Read the model definition and answer for the solid it produces. Units are mm, in the model's axes. A direction names the side the tool comes from. Round coordinates to 2 decimals unless told otherwise and drop trailing zeros. Order: outer loops, then holes, each group sorted by start corner. A loop starts at its lowest first (then second) coordinate and runs counter-clockwise, first axis right, second up.
from build123d import *

# Parameters (mm, degrees)
SKETCH1_R                                         = 8
BOSS_EXTRUDE1_DEPTH                               = 30
SKETCH2_R                                         = 1.5
CUT_EXTRUDE2_DEPTH                                = 30
CSK_FOR_2_FLAT_HEAD_MACHINE_SCREW_100_D           = 2.7051
CSK_FOR_2_FLAT_HEAD_MACHINE_SCREW_100_CSINK_D     = 4.3688
CSK_FOR_2_FLAT_HEAD_MACHINE_SCREW_100_CSINK_ANGLE = 100
CSK_FOR_2_FLAT_HEAD_MACHINE_SCREW_2_D             = 2.7051
CSK_FOR_2_FLAT_HEAD_MACHINE_SCREW_2_CSINK_D       = 4.3688
CSK_FOR_2_FLAT_HEAD_MACHINE_SCREW_2_CSINK_ANGLE   = 100
CSK_FOR_2_FLAT_HEAD_MACHINE_SCREW_3_D             = 2.7051
CSK_FOR_2_FLAT_HEAD_MACHINE_SCREW_3_CSINK_D       = 4.3688
CSK_FOR_2_FLAT_HEAD_MACHINE_SCREW_3_CSINK_ANGLE   = 100
CSK_FOR_2_FLAT_HEAD_MACHINE_SCREW_4_D             = 2.7051
CSK_FOR_2_FLAT_HEAD_MACHINE_SCREW_4_CSINK_D       = 4.3688
CSK_FOR_2_FLAT_HEAD_MACHINE_SCREW_4_CSINK_ANGLE   = 100


with BuildPart() as part:
    # Sketch1 → Boss-Extrude1 (new body)
    with BuildSketch(Plane.XY):
        Polygon((33.27, 7), (31.19936412, 7), (31.19936412, 17), (23.19936412, 17), (19.69936412, 22.18), (13.57063588, 22.18), (10.07063588, 17), (2.07063588, 17), (2.07063588, 7), (0, 7), (0, 0), (33.27, 0), align=None)
        with Locations((16.635, 10.68)):
            Circle(SKETCH1_R, mode=Mode.SUBTRACT)
    extrude(amount=BOSS_EXTRUDE1_DEPTH)

    # Sketch2 → Cut-Extrude2 (cut)
    with BuildSketch(Plane(origin=(0, 17, 0), x_dir=(1, 0, 0), z_dir=(0, 1, 0))):
        with Locations(Location((28.59936412, -6, 0), (0, 0, 270))):
            Circle(SKETCH2_R)
        with Locations(Location((28.59936412, -24, 0), (0, 0, 270))):
            Circle(SKETCH2_R)
        with Locations(Location((4.67063588, -24, 0), (0, 0, 270))):
            Circle(SKETCH2_R)
        with Locations(Location((4.67063588, -6, 0), (0, 0, 270))):
            Circle(SKETCH2_R)
    extrude(amount=-CUT_EXTRUDE2_DEPTH, mode=Mode.SUBTRACT)

    # CSK for _2 Flat Head Machine Screw _100 (through all)
    with Locations(Plane(origin=(0, 17, 0), x_dir=(1, 0, 0), z_dir=(0, 1, 0))):
        with Locations((4.67063588, -6)):
            CounterSinkHole(CSK_FOR_2_FLAT_HEAD_MACHINE_SCREW_100_D / 2, CSK_FOR_2_FLAT_HEAD_MACHINE_SCREW_100_CSINK_D / 2, counter_sink_angle=CSK_FOR_2_FLAT_HEAD_MACHINE_SCREW_100_CSINK_ANGLE)

    # CSK for _2 Flat Head Machine Screw _ 2 (through all)
    with Locations(Plane(origin=(0, 17, 0), x_dir=(1, 0, 0), z_dir=(0, 1, 0))):
        with Locations((4.67063588, -24)):
            CounterSinkHole(CSK_FOR_2_FLAT_HEAD_MACHINE_SCREW_2_D / 2, CSK_FOR_2_FLAT_HEAD_MACHINE_SCREW_2_CSINK_D / 2, counter_sink_angle=CSK_FOR_2_FLAT_HEAD_MACHINE_SCREW_2_CSINK_ANGLE)

    # CSK for _2 Flat Head Machine Screw _ 3 (through all)
    with Locations(Plane(origin=(0, 17, 0), x_dir=(1, 0, 0), z_dir=(0, 1, 0))):
        with Locations((28.59936412, -6)):
            CounterSinkHole(CSK_FOR_2_FLAT_HEAD_MACHINE_SCREW_3_D / 2, CSK_FOR_2_FLAT_HEAD_MACHINE_SCREW_3_CSINK_D / 2, counter_sink_angle=CSK_FOR_2_FLAT_HEAD_MACHINE_SCREW_3_CSINK_ANGLE)

    # CSK for _2 Flat Head Machine Screw _ 4 (through all)
    with Locations(Plane(origin=(0, 17, 0), x_dir=(1, 0, 0), z_dir=(0, 1, 0))):
        with Locations((28.59936412, -24)):
            CounterSinkHole(CSK_FOR_2_FLAT_HEAD_MACHINE_SCREW_4_D / 2, CSK_FOR_2_FLAT_HEAD_MACHINE_SCREW_4_CSINK_D / 2, counter_sink_angle=CSK_FOR_2_FLAT_HEAD_MACHINE_SCREW_4_CSINK_ANGLE)


solid = part.part
Q1. A cutting plane is placed at C-C, the plane z = 12. Give the vertices of the cut face in (x, y) (3 decimals).
Outcome:
outline: (0, 0) - (33.27, 0) - (33.27, 7) - (31.199, 7) - (31.199, 17) - (23.199, 17) - (19.699, 22.18) - (13.571, 22.18) - (10.071, 17) - (2.071, 17) - (2.071, 7) - (0, 7) - close; hole circle Ø16 at (16.635, 10.68)
Q2. Straight lines are drawn through the part: probe 1 along X at (y, z) = (7.25, 24); probe 2 along Z at (x, y) = (6, 2.5); probe 3 along X at (y, z) = (10.75, 15.25). For each, find the intervals that lie inside material, in ascending order.
Outcome:
probe 1: x = 2.07 to 3.17, 6.17 to 9.41, 23.86 to 27.1, 30.1 to 31.2
probe 2: z = 0 to 5.31, 6.69 to 23.31, 24.69 to 30
probe 3: x = 2.07 to 8.64, 24.63 to 31.2
Q3. A cutting plane is placed at A-A, the plane z = 6. Give the vertices of the cut face in (x, y) (3 decimals).
Outcome:
outline: (0, 0) - (3.171, 0) - (3.171, 16.426) - (2.486, 17) - (2.071, 17) - (2.071, 7) - (0, 7) - close; (6.171, 0) - (27.099, 0) - (27.099, 16.426) - (26.415, 17) - (23.199, 17) - (19.699, 22.18) - (13.571, 22.18) - (10.071, 17) - (6.855, 17) - (6.171, 16.426) - close; (30.099, 0) - (33.27, 0) - (33.27, 7) - (31.199, 7) - (31.199, 17) - (30.784, 17) - (30.099, 16.426) - close; hole circle Ø16 at (16.635, 10.68)
Q4. For a pull along Z with two mould halves and no side action, classify faces 1 (the face through (29.61, 8.33, 22.89)), 2 (the face through (24, 6, 30)), 3 (the face through (33.27, 3, 15)) as released by +Z, released by -Z, zero draft, split by the parting line, or undercut.
Outcome:
face 1: undercut
face 2: released by +Z
face 3: zero draft
Q5. A cutting plane is placed at B-B, the plane y = 3.75. Give the vertices of the cut face in (x, z).
Outcome:
outline: (0, 0) - (12.64, 0) - (12.64, 30) - (0, 30) - close; (20.63, 0) - (33.27, 0) - (33.27, 30) - (20.63, 30) - close; hole circle Ø3 at (4.67, 6); hole circle Ø3 at (4.67, 24); hole circle Ø3 at (28.6, 6); hole circle Ø3 at (28.6, 24)
Q6. Flat-ended cylindrical pins translate along their axes: pin 1 (9 mm diameter, centred on x = 5, z = 8.5, fed in from +Y); pin 2 (9 mm diameter, centred on x = 26.5, z = 15, fed in from +Y); pin 3 (3 mm diameter, centred on y = 9.5, z = 21, fed in from -X); pin 4 (2.5 mm diameter, centred on x = 4.67, z = 6, fed in from -Y). Find the tip coordinate at first contact, or state that the pin passes through.
Outcome:
pin 1: stops at y = 17
pin 2: stops at y = 18.78
pin 3: stops at x = 2.07
pin 4: passes through
Q7. A cutting plane is placed at D-D, the plane x = 15. Give the vertices of the cut face in (y, z).
Outcome:
outline: (0, 0) - (2.85, 0) - (2.85, 30) - (0, 30) - close; (18.51, 0) - (22.18, 0) - (22.18, 30) - (18.51, 30) - close
Q8. For faces 4 (the face through (17, 22.18, 15)), 5 (the face through (32, 7, 15)), 6 (the face through (6, 17, 15)), determine the directions among +Z, -Z, +X, -X, +Y, -Y from which every point of the face is accessible in a straight line to the end or side of a thin tool.
Outcome:
face 4: +Z, -Z, +X, -X, +Y
face 5: +Z, -Z, +X, +Y
face 6: +Z, -Z, -X, +Y
